Here's how the part is built. I have some questions about the finished solid (model axes, mm). A direction names the side the tool comes from. Give positions to 0.01 mm unless a question says otherwise; leave off trailing zeros. Loops run counter-clockwise (first coordinate to the right, second up) from the corner with the lowest first, then second, coordinate; pieces in that order, holes last.
Q1. Suppose I cut it at B-B (z = 31). List the corners of the cut face in (x, y) for me, and give its area (3 significant figures).
Q2. Suppose I cut it at A-A (y = 13.5). List the corners of the cut face in (x, z) for me, and give its area (3 significant figures).
Q3. Thinking about a two-plate mould opening in Z: for faces 1 (the face through (0, 25, 25)), 2 (the face through (4, 25, 50)), 3 (the face through (41, 43, 10)), which applies, pulls with the +Z half, pulls with the -Z half, needs draft (parallel to the pull), parting line crosses it, or undercut?
Q4. I need wall thicknesses on probe 1 along X at (y, z) = (45, 19.5); probe 2 along Z at (x, y) = (36, 41.5); probe 3 along Z at (x, y) = (17.5, 3). Which ranges of each line are inside material? Lowest first, please.
Q5. I'm going to push flat-ended pins straight in: P1, Ø16, axis at y = 13.5, z = 28.5, coming from the -X side; P2, Ø12, axis at y = 37.5, z = 41, coming from the +X side; P3, Ø16.5, axis at x = 38.5, y = 42.5, coming from the +Z side. Where does each tip first touch, or does it pass through?
Q6. Suppose I cut it at C-C (x = 19). List the corners of the cut face in (y, z) for me, and give its area (3 significant figures).
Q7. Suppose I cut it at D-D (y = 23). List the corners of the cut face in (x, z) for me, and give its area (3 significant figures).
Q8. For faces 4 (the face through (43.231, 32.913, 40.313)), 5 (the face through (18, 10, 30)), 6 (the face through (30, 0, 19)), 7 (the face through (25, 41, 39)), 8 (the face through (40.569, 42.605, 17.395)), which set-ups out of +Z, -Z, +X, -X, +Y, -Y let a thin tool reach every point of the face, with its end or its side?
```python
from build123d import *

# Parameters (mm, degrees)
F0_W      = 50
F0_H      = 50
F1_DEPTH  = 50
F3_W      = 15
F3_H      = 20
F4_W      = 15
F4_H      = 35.264277
F3_H_2    = 30
F15_DEPTH = 15


with BuildPart() as f1:
    # F0 (on Top) → F1 (new body)
    with BuildSketch(Plane.XY):
        with Locations((25, 25)):
            Rectangle(F0_W, F0_H)
    extrude(amount=F1_DEPTH)

    # F6: sweep along a path in F5
    with BuildLine(Plane.YZ.offset(50)) as f6_path:
        Line((0, 10), (20, 50))
    # F3 (on face) + F4 (on face) → F6 (sweep, cut)
    with BuildSketch(Plane.XY.offset(50)):
        with Locations((17.5, 10)):
            Rectangle(F3_W, F3_H)
    with BuildSketch(Plane.XZ):
        with Locations((17.5, 32.367862)):
            Rectangle(F4_W, F4_H)
    sweep(path=f6_path.line, mode=Mode.SUBTRACT)

    # F8: sweep along a path in F7
    with BuildLine(Plane.YZ.offset(50)) as f8_path:
        Line((50, 10), (20, 50))
    # F3 (on face) → F8 (sweep, cut)
    with BuildSketch(Plane.XY.offset(50)):
        with Locations((17.5, 35)):
            Rectangle(F3_W, F3_H_2)
    sweep(path=f8_path.line, mode=Mode.SUBTRACT)

    # F9: sweep along a path in F5
    with BuildLine(Plane.YZ.offset(50)) as f9_path:
        Line((0, 10), (20, 50))
    # F3 (on face) → F9 (sweep, cut)
    with BuildSketch(Plane.XY.offset(50)):
        Polygon((10, 0), (10, 20), (0, 0), align=None)
    sweep(path=f9_path.line, mode=Mode.SUBTRACT)

    # F10: sweep along a path in F7
    with BuildLine(Plane.YZ.offset(50)) as f10_path:
        Line((50, 10), (20, 50))
    # F3 (on face) → F10 (sweep, cut)
    with BuildSketch(Plane.XY.offset(50)):
        Polygon((10, 50), (0, 50), (10, 20), align=None)
    sweep(path=f10_path.line, mode=Mode.SUBTRACT)

    # F13: sweep along a path in F11
    with BuildLine(Plane.XY.offset(50)) as f13_path:
        Line((25, 50), (50, 0))
    # F12 (on face) → F13 (sweep, cut)
    with BuildSketch(Plane.YZ.offset(50)):
        Polygon((50, 50), (0, 50), (50, 25), align=None)
    sweep(path=f13_path.line, mode=Mode.SUBTRACT)

    # F14 (on face) → F15 (cut)
    with BuildSketch(Plane(origin=(0, 50, 0), x_dir=(-1, 0, 0), z_dir=(0, 1, 0))):
        Polygon((-31.397693, 10), (-50, 25), (-50, 10), align=None)
    extrude(amount=-F15_DEPTH, mode=Mode.SUBTRACT)


solid = f1.part
```
Solutions:
1. outline: (0, 0) - (4.75, 0) - (10, 10.5) - (25, 10.5) - (25, 0) - (50, 0) - (50, 38) - (44, 50) - (25, 50) - (25, 34.25) - (10, 34.25) - (4.75, 50) - (0, 50) - close
1. area: 2,000 mm2
2. outline: (0, 0) - (50, 0) - (50, 43.25) - (43.25, 50) - (25, 50) - (25, 37) - (10, 37) - (6.75, 50) - (0, 50) - close
2. area: 2,260 mm2
3. face 1: needs draft
3. face 2: pulls with the +Z half
3. face 3: undercut
4. probe 1: x = 0 to 9.29, 25 to 43.18
4. probe 2: z = 0 to 10, 13.71 to 43.25
4. probe 3: z = 0 to 16
5. P1: stops at x = 0
5. P2: stops at x = 46.96
5. P3: stops at z = 49.47
6. outline: (0, 0) - (50, 0) - (50, 10) - (20, 50) - (0, 10) - close
6. area: 1,500 mm2
7. outline: (0, 0) - (50, 0) - (50, 38.5) - (38.5, 50) - (25, 50) - (25, 46) - (10, 46) - (9, 50) - (0, 50) - close
7. area: 2,370 mm2
8. face 4: +Z, +X, +Y
8. face 5: +Z, -Y
8. face 6: +Z, -Z, +X, -X, -Y
8. face 7: +Z, +Y
8. face 8: +X, +Y
